Check sheet for the modelled part. Datum: model origin and axes. Units: mm. A direction names the side the tool comes from. Coordinates: 2 decimals unless noted, no trailing zeros. Loops run counter-clockwise (first coordinate to the right, second up) from the corner with the lowest first, then second, coordinate; pieces in that order, holes last. Notation, with made-up numbers: (-36, -30.5) -> (2, -30.5) arc R8 ccw to (2, -19.5) -> close; hole circle Ø10 at (74.5, 46.25). An arc over 180 degrees is marked (long way). Use one line per item in the form item = value.
from build123d import *

# Parameters (mm, degrees)
F1_DEPTH = 30
F2_R     = 0.99999
F2_2_R   = 0.99999
F2_3_R   = 0.99999
F2_4_R   = 0.99999
F3_R     = 40
F4_DEPTH = 2
F5_DEPTH = 25


# Not quite as in the source:
# - a fillet or chamfer is up to 0.001 mm smaller than in the source, because OpenCascade refuses the exact size


with BuildPart() as f1:
    # F0 (on Top) → F1 (new body)
    with BuildSketch(Plane.XY):
        with BuildLine():
            Line((-5.5355339059, 3.5355339059), (-3.5355339059, 3.5355339059))
            ThreePointArc((-3.5355339059, 3.5355339059), (16.4644660941, 23.5355339059), (36.4644660941, 3.5355339059))
            Line((36.4644660941, 3.5355339059), (38.4644660941, 3.5355339059))
            ThreePointArc((38.4644660941, 3.5355339059), (16.4644660941, 25.5355339059), (-5.5355339059, 3.5355339059))
        make_face()
    extrude(amount=F1_DEPTH)

    # F2 (radius 1 in the source; OpenCascade refuses exactly that, so slightly less here)
    f2_edges = [f1.edges().sort_by_distance(p)[0] for p in [
        (-3.535534, 3.535534, 15),
        (-5.535534, 3.535534, 15),
        (38.464466, 3.535534, 15),
        (36.464466, 3.535534, 15),
    ]]
    fillet(f2_edges, radius=F2_R)



with BuildPart() as f1b:
    # F0 (on Top) → F1, piece 2 (new body)
    with BuildSketch(Plane.XY):
        with BuildLine():
            Line((3.5355339059, 5.5355339059), (3.5355339059, 3.5355339059))
            ThreePointArc((3.5355339059, 3.5355339059), (23.5355339059, -16.4644660941), (3.5355339059, -36.4644660941))
            Line((3.5355339059, -36.4644660941), (3.5355339059, -38.4644660941))
            ThreePointArc((3.5355339059, -38.4644660941), (25.5355339059, -16.4644660941), (3.5355339059, 5.5355339059))
        make_face()
    extrude(amount=F1_DEPTH)

    # F2#2 (radius 1 in the source; OpenCascade refuses exactly that, so slightly less here)
    f2_2_edges = [f1b.edges().sort_by_distance(p)[0] for p in [
        (3.535534, 3.535534, 15),
        (3.535534, 5.535534, 15),
        (3.535534, -38.464466, 15),
        (3.535534, -36.464466, 15),
    ]]
    fillet(f2_2_edges, radius=F2_2_R)


with BuildPart() as f1c:
    # F0 (on Top) → F1, piece 3 (new body)
    with BuildSketch(Plane.XY):
        with BuildLine():
            Line((-3.5355339059, -5.5355339059), (-3.5355339059, -3.5355339059))
            ThreePointArc((-3.5355339059, -3.5355339059), (-23.5355339059, 16.4644660941), (-3.5355339059, 36.4644660941))
            Line((-3.5355339059, 36.4644660941), (-3.5355339059, 38.4644660941))
            ThreePointArc((-3.5355339059, 38.4644660941), (-25.5355339059, 16.4644660941), (-3.5355339059, -5.5355339059))
        make_face()
    extrude(amount=F1_DEPTH)

    # F2#4 (radius 1 in the source; OpenCascade refuses exactly that, so slightly less here)
    f2_4_edges = [f1c.edges().sort_by_distance(p)[0] for p in [
        (-3.535534, -3.535534, 15),
        (-3.535534, -5.535534, 15),
        (-3.535534, 38.464466, 15),
        (-3.535534, 36.464466, 15),
    ]]
    fillet(f2_4_edges, radius=F2_4_R)


with BuildPart() as f1d:
    # F0 (on Top) → F1, piece 4 (new body)
    with BuildSketch(Plane.XY):
        with BuildLine():
            Line((5.5355339059, -3.5355339059), (3.5355339059, -3.5355339059))
            ThreePointArc((3.5355339059, -3.5355339059), (-16.4644660941, -23.5355339059), (-36.4644660941, -3.5355339059))
            Line((-36.4644660941, -3.5355339059), (-38.4644660941, -3.5355339059))
            ThreePointArc((-38.4644660941, -3.5355339059), (-16.4644660941, -25.5355339059), (5.5355339059, -3.5355339059))
        make_face()
    extrude(amount=F1_DEPTH)

    # F2#3 (radius 1 in the source; OpenCascade refuses exactly that, so slightly less here)
    f2_3_edges = [f1d.edges().sort_by_distance(p)[0] for p in [
        (3.535534, -3.535534, 15),
        (5.535534, -3.535534, 15),
        (-38.464466, -3.535534, 15),
        (-36.464466, -3.535534, 15),
    ]]
    fillet(f2_3_edges, radius=F2_3_R)


with BuildPart() as f1_1:
    add(f1.part)

    add(f1b.part)  # F4 merges F1b

    add(f1c.part)  # F4 merges F1c

    add(f1d.part)  # F4 merges F1d
    # F3 (on Top) → F4 (join)
    with BuildSketch(Plane.XY):
        Circle(F3_R)
    extrude(amount=-F4_DEPTH)

    # F0 (on Top) → F5 (cut)
    with BuildSketch(Plane.XY):
        Polygon((-3.5355339059, -3.5355339059), (3.5355339059, -3.5355339059), (0, 0), align=None)
        with BuildLine():
            ThreePointArc((-3.5355339059, -3.5355339059), (0, -5), (3.5355339059, -3.5355339059))
            Line((3.5355339059, -3.5355339059), (-3.5355339059, -3.5355339059))
        make_face()
        Polygon((0, 0), (-3.5355339059, 3.5355339059), (-3.5355339059, -3.5355339059), align=None)
        with BuildLine():
            Line((-3.5355339059, -3.5355339059), (-3.5355339059, 3.5355339059))
            ThreePointArc((-3.5355339059, 3.5355339059), (-5, 0), (-3.5355339059, -3.5355339059))
        make_face()
        Polygon((0, 0), (3.5355339059, 3.5355339059), (-3.5355339059, 3.5355339059), align=None)
        with BuildLine():
            Line((-3.5355339059, 3.5355339059), (3.5355339059, 3.5355339059))
            ThreePointArc((3.5355339059, 3.5355339059), (0, 5), (-3.5355339059, 3.5355339059))
        make_face()
        Polygon((3.5355339059, -3.5355339059), (3.5355339059, 3.5355339059), (0, 0), align=None)
        with BuildLine():
            ThreePointArc((3.5355339059, -3.5355339059), (4.6193976626, -1.9134171618), (5, 0))
            ThreePointArc((5, 0), (4.6193976626, 1.9134171618), (3.5355339059, 3.5355339059))
            Line((3.5355339059, 3.5355339059), (3.5355339059, -3.5355339059))
        make_face()
    extrude(amount=-F5_DEPTH, mode=Mode.SUBTRACT)


solid = f1_1.part
(1) Section check C-C, the plane x = 35. Record the boundary of the cut face in (y, z), plus the area to 3 significant figures.
Established:
outline = (-19.36, -2) -> (19.36, -2) -> (19.36, 0) -> (15.39, 0) -> (15.39, 30) -> (11.05, 30) -> (11.05, 0) -> (-19.36, 0) -> close
area = 208 mm²
(2) Tool access check on faces 1 (the flat face through (16, 24, 30)), 2 (the cylindrical face through (-23.53, 16.04, 14.79)). Record the directions out of +Z, -Z, +X, -X, +Y, -Y that give a thin tool (end or side, any length) a straight path to the whole face; none if there is none.
Established:
face_1 = +Z, +X, -X, +Y, -Y
face_2 = +Z
(3) Section check D-D, the plane y = -29. Record the boundary of the cut face in (x, z).
Established:
outline = (-27.55, -2) -> (27.55, -2) -> (27.55, 0) -> (21.61, 0) -> (21.61, 30) -> (19.12, 30) -> (19.12, 0) -> (-27.55, 0) -> close
(4) Scan lines: line 1 along X through (y, z) = (11.5, 2.5); line 2 along X through (y, z) = (-9, 11.5); line 3 along Y through (x, z) = (11, 22.5). Record each from-to range of solid material in increasing order.
Established:
line_1 = -24.97 to -22.91, -4.04 to -1.88, 34.81 to 36.97
line_2 = -37.78 to -35.7, 2.77 to 4.85, 22.09 to 24.23
line_3 = -37.16 to -35.02, 2.09 to 4.23, 22.77 to 24.85
(5) Mould release check, pull along X, two halves, no side actions. Record for faces 3 (the cylindrical face through (-16.04, -23.53, 14.79)), 4 (the cylindrical face through (16.04, 23.53, 14.79)), 5 (the flat face through (8, 1, -2)), 6 (the cylindrical face through (-8.67, -39.05, -0.99)): +X half, -X half, draft (parallel to the pull), parting line (faces both ways), or undercut.
Established:
face_3 = undercut
face_4 = undercut
face_5 = draft
face_6 = parting line
(6) Go/stop test with flat-tipped pins: P1, Ø5, axis at x = -1, y = 24.5, coming from the +Z side; P2, Ø12, axis at y = 0, z = 10.5, coming from the -X side; P3, Ø1.5, axis at y = 3.5, z = 22, coming from the +X side. Record where each tip stops, or that it passes through.
Established:
P1 = 0
P2 = -38.44
P3 = 38.4
(7) Section check B-B, the plane x = 0. Record the boundary of the cut face in (y, z).
Established:
outline = (-40, -2) -> (-5, -2) -> (-5, 0) -> (-14.89, 0) -> (-14.89, 30) -> (-18.13, 30) -> (-18.13, 0) -> (-40, 0) -> close; (5, -2) -> (40, -2) -> (40, 0) -> (18.13, 0) -> (18.13, 30) -> (14.89, 30) -> (14.89, 0) -> (5, 0) -> close
(8) Section check A-A, the plane z = 25. Give the number of separate pieces and of enclosed holes in the cut face, plus the area to 3 significant figures.
Established:
separate_pieces = 4
enclosed_holes = 0
area = 524 mm²
